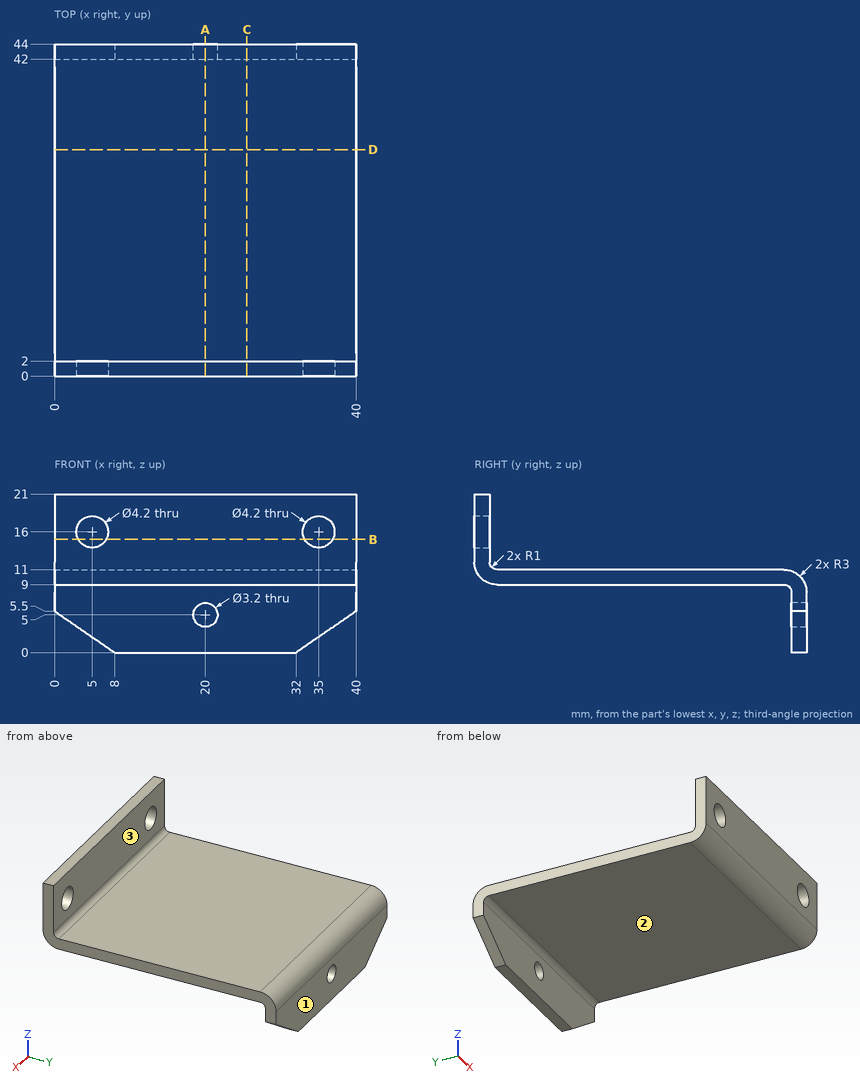
Input: dimensioned drawing with shaded views. Units: mm. Origin: part minimum x, y, z. A direction names the side the tool comes from. Round coordinates to 2 decimals unless told otherwise and drop trailing zeros. Loops run counter-clockwise (first coordinate to the right, second up) from the corner with the lowest first, then second, coordinate; pieces in that order, holes last. Notation, with made-up numbers: (-27.75, -25) -> (-14.75, -25) arc R28 cw to (-14.75, 2) -> close; hole circle Ø7 at (-8.75, 31). An arc over 180 degrees is marked (long way). Answer as a JSON object with one key per item and string values. Group by question number.
Q1. Section query A-A (x = 20). Output: boundary loops of the cut face in (y, z), plus the area to 3 significant figures.
Q2. Section query B-B (z = 15). Output: boundary loops of the cut face in (x, y).
Q3. Section query D-D (y = 30). Output: boundary loops of the cut face in (x, z).
Q4. Access query for the marked faces 1, 2 and 3. Directions: +Z, -Z, +X, -X, +Y, -Y. A direction counts if a zero-diameter tool reaches every point of the face in a straight line with its end or side. Return the directions, or none.
Q5. Ray query, line 1 (X direction, y = 1, z = 16); line 2 (Y direction, x = 15, z = 3.25); line 3 (Z direction, x = 12.5, y = 22). Return the intervals inside material, ascending. Write a range as from..to.
Q6. Section query C-C (x = 25.5). Output: boundary loops of the cut face in (y, z), plus the area to 3 significant figures.
Q7. Contact query for flat-ended pins moving along their axis: P1, Ø10, axis at x = 34.5, y = 33.5, coming from the +Z side; P2, Ø5.5, axis at x = 35, z = 16, coming from the +Y side; P3, Ø5, axis at x = 9.5, z = 13, coming from the -Y side; P4, Ø4, axis at x = 12, z = 5, coming from the -Y side. Output: stop coordinate, or through.
Completed:
{
 "1": {"outline": "(0, 12) arc R3 ccw to (3, 9) -> (41, 9) arc R1 cw to (42, 8) -> (42, 6.6) -> (44, 6.6) -> (44, 8) arc R3 ccw to (41, 11) -> (3, 11) arc R1 cw to (2, 12) -> (2, 21) -> (0, 21) -> close; (42, 0) -> (44, 0) -> (44, 3.4) -> (42, 3.4) -> close", "area": "116 mm²"},
 "2": {"outline": "(0, 0) -> (3.15, 0) -> (3.15, 2) -> (0, 2) -> close; (6.85, 0) -> (33.15, 0) -> (33.15, 2) -> (6.85, 2) -> close; (36.85, 0) -> (40, 0) -> (40, 2) -> (36.85, 2) -> close"},
 "3": {"outline": "(0, 9) -> (40, 9) -> (40, 11) -> (0, 11) -> close"},
 "4": {"face 1": "+Z, -Z, +X, -X, +Y", "face 2": "-Z, +X, -X, -Y", "face 3": "+Z, +X, -X, +Y"},
 "5": {"line 1": "0..2.9, 7.1..32.9, 37.1..40", "line 2": "42..44", "line 3": "9..11"},
 "6": {"outline": "(0, 12) arc R3 ccw to (3, 9) -> (41, 9) arc R1 cw to (42, 8) -> (42, 0) -> (44, 0) -> (44, 8) arc R3 ccw to (41, 11) -> (3, 11) arc R1 cw to (2, 12) -> (2, 21) -> (0, 21) -> close", "area": "123 mm²"},
 "7": {"P1": "z = 11", "P2": "y = 2", "P3": "y = 0", "P4": "y = 42"}
}
